```python
from build123d import *

# Parameters (mm, degrees)
SKETCH1_W           = 160
SKETCH1_H           = 57
SKETCH1_R           = 30
SKETCH1_W_2         = 105
SKETCH1_H_2         = 108
BOSS_EXTRUDE1_DEPTH = 15
CUT_EXTRUDE1_START  = -572.5
SKETCH2_W           = 20
SKETCH2_H           = 10
CUT_EXTRUDE1_DEPTH  = 497.5
CUT_EXTRUDE2_START  = -677.5
SKETCH2_3_W         = 20
SKETCH2_3_H         = 10
CUT_EXTRUDE2_DEPTH  = 973.5
CUT_EXTRUDE3_START  = 13
SKETCH1_3_W         = 105
SKETCH1_3_H         = 108
CUT_EXTRUDE3_DEPTH  = 3
CUT_EXTRUDE4_START  = -572.5
SKETCH2_4_W         = 20
SKETCH2_4_H         = 10
CUT_EXTRUDE4_DEPTH  = 497.5
CUT_EXTRUDE5_START  = -1250
SKETCH2_5_W         = 20
SKETCH2_5_H         = 10
CUT_EXTRUDE5_DEPTH  = 572.5
SKETCH4_W           = 20
SKETCH4_H           = 20
CUT_EXTRUDE6_DEPTH  = 5
SKETCH3_W           = 20
SKETCH3_H           = 600
CUT_EXTRUDE7_DEPTH  = 10


with BuildPart() as part:
    # Sketch1 → Boss-Extrude1 (new body)
    with BuildSketch(Plane(origin=(0, 0, 0), x_dir=(1, 0, 0), z_dir=(0, 1, 0))):
        Polygon((-825, 375), (-825, -375), (825, -375), (825, 375), (-147.5, 375), (-147.5, 267), (-252.5, 267), (-252.5, 375), align=None)
        with Locations((-482.5, 295)):
            Rectangle(SKETCH1_W, SKETCH1_H, mode=Mode.SUBTRACT)
        with Locations((325, 295)):
            Circle(SKETCH1_R, mode=Mode.SUBTRACT)
        with Locations((-200, 321)):
            Rectangle(SKETCH1_W_2, SKETCH1_H_2)
    extrude(amount=BOSS_EXTRUDE1_DEPTH)

    # Sketch2 → Cut-Extrude1 (cut)
    with BuildSketch(Plane.ZY.offset(825).offset(CUT_EXTRUDE1_START)):
        with Locations((-337.5, 5)):
            Rectangle(SKETCH2_W, SKETCH2_H)
    extrude(amount=CUT_EXTRUDE1_DEPTH, mode=Mode.SUBTRACT)

    # Sketch2<3> → Cut-Extrude2 (cut, through all)
    with BuildSketch(Plane.ZY.offset(825).offset(CUT_EXTRUDE2_START)):
        with Locations((-337.5, 5)):
            Rectangle(SKETCH2_3_W, SKETCH2_3_H)
    extrude(amount=-CUT_EXTRUDE2_DEPTH, mode=Mode.SUBTRACT)

    # Sketch1<3> → Cut-Extrude3 (cut, through all)
    with BuildSketch(Plane(origin=(0, 0, 0), x_dir=(1, 0, 0), z_dir=(0, 1, 0)).offset(CUT_EXTRUDE3_START)):
        with Locations((-200, 321)):
            Rectangle(SKETCH1_3_W, SKETCH1_3_H)
    extrude(amount=CUT_EXTRUDE3_DEPTH, mode=Mode.SUBTRACT)

    # Sketch2<4> → Cut-Extrude4 (cut)
    with BuildSketch(Plane.ZY.offset(825).offset(CUT_EXTRUDE4_START)):
        with Locations((337.5, 5)):
            Rectangle(SKETCH2_4_W, SKETCH2_4_H)
    extrude(amount=CUT_EXTRUDE4_DEPTH, mode=Mode.SUBTRACT)

    # Sketch2<5> → Cut-Extrude5 (cut)
    with BuildSketch(Plane.ZY.offset(825).offset(CUT_EXTRUDE5_START)):
        with Locations((337.5, 5)):
            Rectangle(SKETCH2_5_W, SKETCH2_5_H)
    extrude(amount=CUT_EXTRUDE5_DEPTH, mode=Mode.SUBTRACT)

    # Sketch4 → Cut-Extrude6 (cut)
    with BuildSketch(Plane.XZ):
        with Locations((-242.5, -337.5)):
            Rectangle(SKETCH4_W, SKETCH4_H)
        with Locations((-157.5, -337.5)):
            Rectangle(SKETCH4_W, SKETCH4_H)
        with Locations((-157.5, 337.5)):
            Rectangle(SKETCH4_W, SKETCH4_H)
        with Locations((-242.5, 337.5)):
            Rectangle(SKETCH4_W, SKETCH4_H)
    extrude(amount=-CUT_EXTRUDE6_DEPTH, mode=Mode.SUBTRACT)

    # Sketch3 → Cut-Extrude7 (cut)
    with BuildSketch(Plane.XZ):
        with Locations((-787.5, 0)):
            Rectangle(SKETCH3_W, SKETCH3_H)
    extrude(amount=-CUT_EXTRUDE7_DEPTH, mode=Mode.SUBTRACT)


solid = part.part
```
Input: part model. Units: mm. Frame: model coordinates. Give positions to 0.01 mm unless a question says otherwise; leave off trailing zeros. Order: outer loops, then holes, each group sorted by start corner. A loop starts at its lowest first (then second) coordinate and runs counter-clockwise, first axis right, second up. Notation, with made-up numbers: M 9.5,78 L 15.5,78 A9 cw 15.5,94 Z; hole C 32.5,50.25 d8. An arc over 180 degrees is marked long. Return JSON: item names as keys, results as strings.
1) Section query B-B on x = -63. Output: boundary loops of the cut face in (y, z), and give its area (4 significant figures).
Taken from the geometry:
{"outline": "M 0,-375 L 15,-375 L 15,375 L 0,375 L 0,347.5 L 10,347.5 L 10,327.5 L 0,327.5 L 0,-327.5 L 10,-327.5 L 10,-347.5 L 0,-347.5 Z", "area": "10,850 mm2"}
2) Contact query for flat-ended pins moving along their axis: pin 1 (16 mm diameter, centred on x = 274, z = 334, fed in from -Y); pin 2 (1.6 mm diameter, centred on x = -175.5, y = 14, fed in from -Z); pin 3 (16 mm diameter, centred on x = -247, z = 338.5, fed in from -Y). Output: stop coordinate, or through.
Taken from the geometry:
{"pin 1": "stops at y = 0", "pin 2": "stops at z = -267", "pin 3": "stops at y = 5"}
3) Line query: L1, parallel to X at y = 9.25, z = -295; L2, parallel to X at y = 5.5, z = 340; L3, parallel to Z at x = 325, y = 3.5. Output: solid intervals per line, ascending. Write a range as [from, to].
Taken from the geometry:
{"L1": "x = [-825, -797.5], [-777.5, -562.5], [-402.5, 295], [355, 825]", "L2": "x = [-825, -750], [-252.5, -147.5], [425, 825]", "L3": "z = [-375, -347.5], [-327.5, -325], [-265, 327.5], [347.5, 375]"}
4) Mould query, pull axis X, two halves, no side actions, for faces 1 (the face through (-12, 15, -5)), 2 (the face through (301, 7, -277)), 3 (the face through (-201, 13, -322)). Classes: released by +X, released by -X, zero draft, split by the parting line, or undercut.
Taken from the geometry:
{"face 1": "zero draft", "face 2": "undercut", "face 3": "undercut"}
5) Section query A-A on x = 325. Output: boundary loops of the cut face in (y, z), and give its area (3 significant figures).
Taken from the geometry:
{"outline": "M 0,-375 L 15,-375 L 15,-325 L 0,-325 L 0,-327.5 L 10,-327.5 L 10,-347.5 L 0,-347.5 Z; M 0,-265 L 15,-265 L 15,375 L 0,375 L 0,347.5 L 10,347.5 L 10,327.5 L 0,327.5 Z", "area": "9,950 mm2"}
